```python
from build123d import *

# Parameters (mm, degrees)
F0_W        = 20.32
F0_H        = 38.1
F1_DEPTH    = 20.32
F2_SIZE2    = 6.8059094878
F2_SIZE     = 25.4
F2_2_SIZE2  = 6.8059094878
F2_2_SIZE   = 25.4
F3_R        = 5.715
F4_DEPTH    = 25.4
F5_W        = 68.5800006613
F5_H        = 10.5876065791
F6_DEPTH    = 35.56
F7_R        = 7.9375
F8_DEPTH    = 12.7
F9_T1_DEPTH = 46.99
F9_T3_DEPTH = 54.5211276147
F9_T5_DEPTH = 34.9846968374
F9_T7_DEPTH = 23.6639734387


# Not quite as in the source:
# - a fillet or chamfer that OpenCascade refuses, or shapes differently, is made with other operations: its cross-section is extruded or revolved along the edge and cut away or added


with BuildPart() as f1:
    # F0 (on Right) → F1 (new body)
    with BuildSketch(Plane.YZ):
        with Locations((-27.8230281547, -4.4044164286)):
            Rectangle(F0_W, F0_H)
    extrude(amount=F1_DEPTH)

    # F2
    f2_edges = [f1.edges().sort_by_distance(p)[0] for p in [
        (20.32, -27.823028, -23.454416),
    ]]
    f2_side = f1.faces().sort_by_distance((20.32, -27.823028, -4.404416))[0]
    chamfer(f2_edges, length=F2_SIZE, length2=F2_SIZE2, reference=f2_side)

    # F2#2
    f2_2_edges = [f1.edges().sort_by_distance(p)[0] for p in [
        (0, -27.823028, -23.454416),
    ]]
    f2_2_side = f1.faces().sort_by_distance((0, -27.823028, -4.404416))[0]
    chamfer(f2_2_edges, length=F2_2_SIZE, length2=F2_2_SIZE2, reference=f2_2_side)

    # F3 (on face) → F4 (cut)
    with BuildSketch(Plane.XZ.offset(37.9830281547)):
        with Locations((10.16, 1.2867113903)):
            Circle(F3_R)
    extrude(amount=-F4_DEPTH, mode=Mode.SUBTRACT)

    # F5 (on face) → F6 (cut)
    with BuildSketch(Plane(origin=(18.4724222096, 0, -4.9496706133), x_dir=(0, 1, 0), z_dir=(0.9659258263, 0, -0.2588190451))):
        with Locations((-23.6119744368, -18.386438489)):
            Rectangle(F5_W, F5_H)
    extrude(amount=-F6_DEPTH, mode=Mode.SUBTRACT)

    # F7 (on face) → F8 (join)
    with BuildSketch(Plane.XY.offset(14.6455835714)):
        with Locations((10.16, -27.8230281547)):
            Circle(F7_R)
    extrude(amount=F8_DEPTH)

    # F9: fillet of radius 5.08 on 8 edges, made by hand

    # F9_s2 → F9_t1 (cut)
    with BuildSketch(Plane.XY.offset(-19.6444164286)):
        with BuildLine():
            ThreePointArc((20.32, -22.7430281547), (18.8321024484, -19.1509257062), (15.24, -17.6630281547))
            Line((15.24, -17.6630281547), (20.32, -17.6630281547))
            Line((20.32, -17.6630281547), (20.32, -22.7430281547))
        make_face()
        with BuildLine():
            ThreePointArc((0, -22.7430281547), (1.4878975516, -19.1509257062), (5.08, -17.6630281547))
            Line((5.08, -17.6630281547), (0, -17.6630281547))
            Line((0, -17.6630281547), (0, -22.7430281547))
        make_face()
        with BuildLine():
            ThreePointArc((5.08, -37.9830281547), (1.4878975516, -36.4951306031), (0, -32.9030281547))
            Line((0, -32.9030281547), (0, -37.9830281547))
            Line((0, -37.9830281547), (5.08, -37.9830281547))
        make_face()
        with BuildLine():
            ThreePointArc((15.24, -37.9830281547), (18.8321024484, -36.4951306031), (20.32, -32.9030281547))
            Line((20.32, -32.9030281547), (20.32, -37.9830281547))
            Line((20.32, -37.9830281547), (15.24, -37.9830281547))
        make_face()
    extrude(amount=F9_T1_DEPTH, mode=Mode.SUBTRACT)

    # F9_s4 → F9_t3 (cut)
    with BuildSketch(Plane(origin=(7.4354809742, 0, 27.7495927742), x_dir=(0, 1, 0), z_dir=(-0.2588190451, 0, -0.9659258263))):
        with BuildLine():
            ThreePointArc((-37.9830281547, 14.0440587081), (-36.4951306031, 17.6361611565), (-32.9030281547, 19.1240587081))
            Line((-32.9030281547, 19.1240587081), (-37.9830281547, 19.1240587081))
            Line((-37.9830281547, 19.1240587081), (-37.9830281547, 14.0440587081))
        make_face()
        with BuildLine():
            ThreePointArc((-22.7430281547, 19.1240587081), (-19.1509257062, 17.6361611565), (-17.6630281547, 14.0440587081))
            Line((-17.6630281547, 14.0440587081), (-17.6630281547, 19.1240587081))
            Line((-17.6630281547, 19.1240587081), (-22.7430281547, 19.1240587081))
        make_face()
    extrude(amount=F9_T3_DEPTH, mode=Mode.SUBTRACT)

    # F9_s6 → F9_t5 (cut)
    with BuildSketch(Plane.XZ.offset(10.330679736)):
        with BuildLine():
            ThreePointArc((7.3074886766, -15.5125290504), (5.0301869773, -14.1977283012), (3.7153862282, -11.9204266019))
            Line((3.7153862282, -11.9204266019), (4.4744867946, -14.7534284839))
            Line((4.4744867946, -14.7534284839), (7.3074886766, -15.5125290504))
        make_face()
    extrude(amount=F9_T5_DEPTH, mode=Mode.SUBTRACT)

    # F9_s8 → F9_t7 (cut)
    with BuildSketch(Plane.XZ.offset(15.9910414353)):
        with BuildLine():
            ThreePointArc((0, 2.6143782591), (0.0434601042, 1.9513052026), (0.1730968025, 1.29957751))
            Line((0.1730968025, 1.29957751), (0, 1.9455835714))
            Line((0, 1.9455835714), (0, 2.6143782591))
        make_face()
    extrude(amount=F9_T7_DEPTH, mode=Mode.SUBTRACT)


solid = f1.part
```
Source: CAD feature listing. Evaluate the final solid. Frame: model axes, mm. A direction names the side the tool comes from. Coordinates: 2 decimals unless noted, no trailing zeros. Order: outer loops, then holes, each group sorted by start corner. A loop starts at its lowest first (then second) coordinate and runs counter-clockwise, first axis right, second up. Notation, with made-up numbers: (22.5, 2) - (55.5, 2) arc R26 ccw to (55.5, 20) - close; hole circle Ø9 at (-40, 43). An arc over 180 degrees is marked (long way). One line per item, written item: value.
1) Cut plane B-B on y = -29.25. Output: boundary loops of the cut face in (x, z) (3 decimals), plus the area to 3 significant figures.
Computed values:
outline: (0, 2.614) arc R5.08 ccw to (0.173, 1.3) - (3.715, -11.92) arc R5.08 ccw to (7.307, -15.513) - (15.084, -17.596) - (20.32, 1.946) - (20.32, 14.646) - (17.968, 14.646) - (17.968, 27.346) - (2.352, 27.346) - (2.352, 14.646) - (0, 14.646) - close; hole circle Ø11.43 at (10.16, 1.287)
area: 633 mm^2
2) Ray query, line 1 (Z direction, x = 10.16, y = -31.75); line 2 (X direction, y = -24, z = 4); line 3 (Z direction, x = 14.5, y = -27.75) (3 decimals). Return the intervals inside material, ascending. Write a range as [from, to].
Computed values:
line 1: z = [-16.28, -4.43], [7, 27.35]
line 2: x = [0, 5.13], [15.19, 20.32]
line 3: z = [-17.44, -2.432], [5.005, 27.346]
3) Mould query, pull axis Z, two halves, no side actions, for faces 3 (the face through (14.43, -21.13, 20.91)), 4 (the face through (5.057, -27.681, -14.224)), 5 (the face through (15.611, -27.965, 3.003)). Classes: released by +Z, released by -Z, zero draft, split by the parting line, or undercut.
Computed values:
face 3: zero draft
face 4: released by -Z
face 5: undercut
4) Cut plane C-C on x = 9.5. Output: boundary loops of the cut face in (y, z).
Computed values:
outline: (-37.98, -16.1) - (-17.66, -16.1) - (-17.66, -4.39) - (-37.98, -4.39) - close; (-37.98, 6.96) - (-17.66, 6.96) - (-17.66, 14.65) - (-19.91, 14.65) - (-19.91, 27.35) - (-35.73, 27.35) - (-35.73, 14.65) - (-37.98, 14.65) - close
5) Cut plane A-A on z = 5. Output: boundary loops of the cut face in (x, y), plus the area to 3 significant figures.
Computed values:
outline: (0, -32.9) arc R5.08 ccw to (5.08, -37.98) - (5.82, -37.98) - (5.82, -17.66) - (5.08, -17.66) arc R5.08 ccw to (0, -22.74) - close; (14.5, -37.98) - (15.24, -37.98) arc R5.08 ccw to (20.32, -32.9) - (20.32, -22.74) arc R5.08 ccw to (15.24, -17.66) - (14.5, -17.66) - close
area: 214 mm^2
6) Reachability of faces 1 (the face through (0, -28, 9)), 2 (the face through (3, -23, 14.646)) from +Z, -Z, +X, -X, +Y, -Y: full face, straight path, thin tool, end or side. Return the list, or none.
Computed values:
face 1: +Z, -Z, -X, +Y, -Y
face 2: +Z
7) Cut plane D-D on z = 13. Output: boundary loops of the cut face in (x, y).
Computed values:
outline: (0, -32.9) arc R5.08 ccw to (5.08, -37.98) - (15.24, -37.98) arc R5.08 ccw to (20.32, -32.9) - (20.32, -22.74) arc R5.08 ccw to (15.24, -17.66) - (5.08, -17.66) arc R5.08 ccw to (0, -22.74) - close
8) Contact query for flat-ended pins moving along their axis: pin 1 (4 mm diameter, centred on y = -22, z = -9.5, fed in from +X); pin 2 (6 mm diameter, centred on y = -29, z = -7, fed in from -X); pin 3 (5 mm diameter, centred on y = -33, z = -12, fed in from +X); pin 4 (9 mm diameter, centred on x = 10.16, z = 1.29, fed in from +Y). Output: stop coordinate, or through.
Computed values:
pin 1: stops at x = 17.77
pin 2: stops at x = 1.59
pin 3: stops at x = 17.25
pin 4: passes through
